Work out the finished part from the listing and answer in its coordinate system (mm). Face numbers are marked on the shaded views. A direction names the side the tool comes from. Round coordinates to 2 decimals unless told otherwise and drop trailing zeros. Loops run counter-clockwise (first coordinate to the right, second up) from the corner with the lowest first, then second, coordinate; pieces in that order, holes last. Notation, with made-up numbers: M 74.25,-12 L 120.25,-12 A12 ccw 120.25,7 Z; hole C -35.75,28.25 d1. An arc over 180 degrees is marked long. One line per item, written item: value.
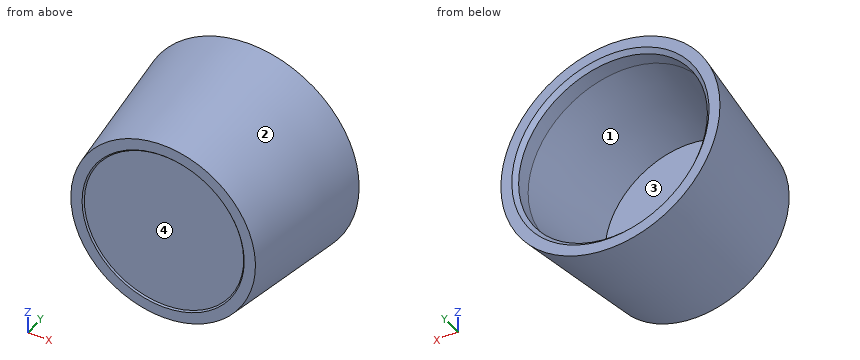
```python
from build123d import *

# Parameters (mm, degrees)
CHAMFER1_SIZE = 1.905


with BuildPart() as part:
    # Sketch1 → Revolve1 (revolve)
    with BuildSketch(Plane(origin=(0, 0, 0), x_dir=(0, 0, -1), z_dir=(1, 0, 0))):
        Polygon((41.733180383, 0), (49.53, 63.5), (42.680526601, 63.5), (42.680526601, 54.61), (36.910880084, 7.62), (0, 7.62), (0, 0.635), (36.018180383, 0.635), (36.653180383, 0), align=None)
    revolve(axis=Axis((0, 0, 0), (0, 1, 0)))

    # Chamfer1
    chamfer1_edges = [part.edges().sort_by_distance(p)[0] for p in [
        (0, 63.5, 42.680526601),
    ]]
    chamfer(chamfer1_edges, length=CHAMFER1_SIZE)


solid = part.part
```
1) For the marked faces 3 and 4, determine the directions among +Z, -Z, +X, -X, +Y, -Y from which every point of the face is accessible in a straight line to the end or side of a thin tool.
Check values:
face 3: +Y
face 4: -Y
2) Find the intervals of material crossed by probe 1 along Y at (x, z) = (26, 14) (3 decimals); probe 2 along X at (y, z) = (58, 0); probe 3 along X at (y, z) = (19, -4.5), in increasing order. Write a range as from..to.
Check values:
probe 1: 0.635..7.62
probe 2: -48.85..-42.68, 42.68..48.85
probe 3: -43.84..-38.04, 38.04..43.84
3) Find section A-A (x = 0). Give the vertices of the cut face in (y, z) (3 decimals).
Check values:
outline: M 0,-41.733 L 63.5,-49.53 L 63.5,-44.586 L 61.595,-42.681 L 54.61,-42.681 L 7.62,-36.911 L 7.62,36.911 L 54.61,42.681 L 61.595,42.681 L 63.5,44.586 L 63.5,49.53 L 0,41.733 L 0,36.653 L 0.635,36.018 L 0.635,-36.018 L 0,-36.653 Z
4) Find section B-B (z = 0). Give the vertices of the cut face in (x, y) (3 decimals).
Check values:
outline: M -49.53,63.5 L -41.733,0 L -36.653,0 L -36.018,0.635 L 36.018,0.635 L 36.653,0 L 41.733,0 L 49.53,63.5 L 44.586,63.5 L 42.681,61.595 L 42.681,54.61 L 36.911,7.62 L -36.911,7.62 L -42.681,54.61 L -42.681,61.595 L -44.586,63.5 Z
5) Find section D-D (y = 9.5). Give the vertices of the cut face in (x, z), then the cut area to 3 significant figures.
Check values:
outline: C 0,0 d85.8; hole C 0,0 d74.28
area: 1,450 mm2
6) Find section C-C (y = 43.5). Give the vertices of the cut face in (x, z).
Check values:
outline: C 0,0 d94.15; hole C 0,0 d82.63
7) Each of these flat-tipped pins is pushed along its axis until it touches: pin 1 (12 mm diameter, centred on x = -22.5, z = 12.5, fed in from +Y); pin 2 (3 mm diameter, centred on y = 48.5, z = 21.5, fed in from +X); pin 3 (12 mm diameter, centred on x = -12, z = 2.5, fed in from -Y) (3 decimals). Where does it stop, or does it pass through?
Check values:
pin 1: y = 7.62
pin 2: x = 43.32
pin 3: y = 0.635
8) The mould has two halves that part along X. Classify the marked faces 1 and 2: +X half, -X half, draft (parallel to the pull), parting line (faces both ways), or undercut.
Check values:
face 1: undercut
face 2: parting line
